Geometry check sheet. Reference: the model listing, model coordinates, mm. A direction names the side the tool comes from. Give positions to 0.01 mm unless a question says otherwise; leave off trailing zeros. Loops run counter-clockwise (first coordinate to the right, second up) from the corner with the lowest first, then second, coordinate; pieces in that order, holes last. Notation, with made-up numbers: (17, 89.5) -> (47, 89.5) arc R9 cw to (47, 95.5) -> close; hole circle Ø11 at (36.25, -24.5). An arc over 180 degrees is marked (long way). Answer as a JSON object with one key per item and string values.
from build123d import *

# Parameters (mm, degrees)
F2_R     = 12
F3_DEPTH = 20


with BuildPart() as f1:
    # F0 (on Front) → F1 (revolve)
    with BuildSketch(Plane.XZ):
        Polygon((40, 33), (40, 0), (45, 0), (45, 3), (75, 3), (75, 23), (45, 23), (45, 33), align=None)
    revolve(axis=Axis((0, 0, 39.782755), (0, 0, 1)))

    # F2 (on face) → F3 (cut, through all)
    with BuildSketch(Plane.XY.offset(23)):
        with Locations((0, 60)):
            Circle(F2_R)
        with Locations((-57.063391, 18.54102)):
            Circle(F2_R)
        with Locations((-35.267115, -48.54102)):
            Circle(F2_R)
        with Locations((35.267115, -48.54102)):
            Circle(F2_R)
        with Locations((57.063391, 18.54102)):
            Circle(F2_R)
    extrude(amount=-F3_DEPTH, mode=Mode.SUBTRACT)


solid = f1.part
1) Draft check along X on faces 1 (the face through (-9.764, 74.362, 13.14)), 2 (the face through (-29.73, -59.187, 13.14)), 3 (the face through (48.22, 26.65, 13.14)), 4 (the face through (-30.2, -26.5, 33)). Enter one of: pulls with the +X half, pulls with the -X half, needs draft (parallel to the pull), parting line crosses it, or undercut.
Geometry check:
{"face 1": "parting line crosses it", "face 2": "undercut", "face 3": "undercut", "face 4": "needs draft"}
2) Section check C-C on y = -42.5. Record the cut outline in (x, z).
Geometry check:
{"outline": "(-61.8, 3) -> (-45.64, 3) -> (-45.64, 23) -> (-61.8, 23) -> close; (-24.9, 3) -> (-14.79, 3) -> (-14.79, 0) -> (14.79, 0) -> (14.79, 3) -> (24.9, 3) -> (24.9, 23) -> (14.79, 23) -> (14.79, 33) -> (-14.79, 33) -> (-14.79, 23) -> (-24.9, 23) -> close; (45.64, 3) -> (61.8, 3) -> (61.8, 23) -> (45.64, 23) -> close"}
3) Depth check by flat-ended pin: P1, Ø4, axis at y = -3, z = 26.5, coming from the -X side; P2, Ø12, axis at y = -33.5, z = 4.5, coming from the +X side; P3, Ø10, axis at x = 43.5, y = 47, coming from the -Z side. Enter the tip coordinate at first touch or a pass-through.
Geometry check:
{"P1": "stops at x = -44.99", "P2": "stops at x = 69.78", "P3": "stops at z = 3"}
4) Tool access check on faces 5 (the face through (20.765, -39.923, 28.07)), 6 (the face through (20.765, -39.923, 1.521)), 7 (the face through (-2.601, 48.285, 13.14)). Record the directions out of +Z, -Z, +X, -X, +Y, -Y that give a thin tool (end or side, any length) a straight path to the whole face; none if there is none.
Geometry check:
{"face 5": "+Z", "face 6": "-Z", "face 7": "+Z, -Z"}
5) Section check B-B on y = 60. Record the cut outline in (x, z).
Geometry check:
{"outline": "(-45, 3) -> (-12, 3) -> (-12, 23) -> (-45, 23) -> close; (12, 3) -> (45, 3) -> (45, 23) -> (12, 23) -> close"}
6) Material ranges on line 1 along Y through (x, z) = (0, 13); line 2 along X through (y, z) = (-46, 16.5) (3 decimals); line 3 along X through (y, z) = (12, 5.5), recorded low to high. Write a range as from..to.
Geometry check:
{"line 1": "y = -75..-40, 40..48, 72..75", "line 2": "x = -59.237..-46.995, -23.539..23.539, 46.995..59.237", "line 3": "x = -74.03..-67.12, -47..-38.16, 38.16..47, 67.12..74.03"}
7) Section check A-A on x = 0. Record the cut outline in (y, z), plus the area to 3 significant figures.
Geometry check:
{"outline": "(-75, 3) -> (-45, 3) -> (-45, 0) -> (-40, 0) -> (-40, 33) -> (-45, 33) -> (-45, 23) -> (-75, 23) -> close; (40, 0) -> (45, 0) -> (45, 3) -> (48, 3) -> (48, 23) -> (45, 23) -> (45, 33) -> (40, 33) -> close; (72, 3) -> (75, 3) -> (75, 23) -> (72, 23) -> close", "area": "1,050 mm2"}
8) Section check D-D on x = -15. Record the cut outline in (y, z), plus the area to 3 significant figures.
Geometry check:
{"outline": "(-73.48, 3) -> (-42.43, 3) -> (-42.43, 0) -> (-37.08, 0) -> (-37.08, 33) -> (-42.43, 33) -> (-42.43, 23) -> (-73.48, 23) -> close; (37.08, 0) -> (42.43, 0) -> (42.43, 3) -> (73.48, 3) -> (73.48, 23) -> (42.43, 23) -> (42.43, 33) -> (37.08, 33) -> close", "area": "1,600 mm2"}
